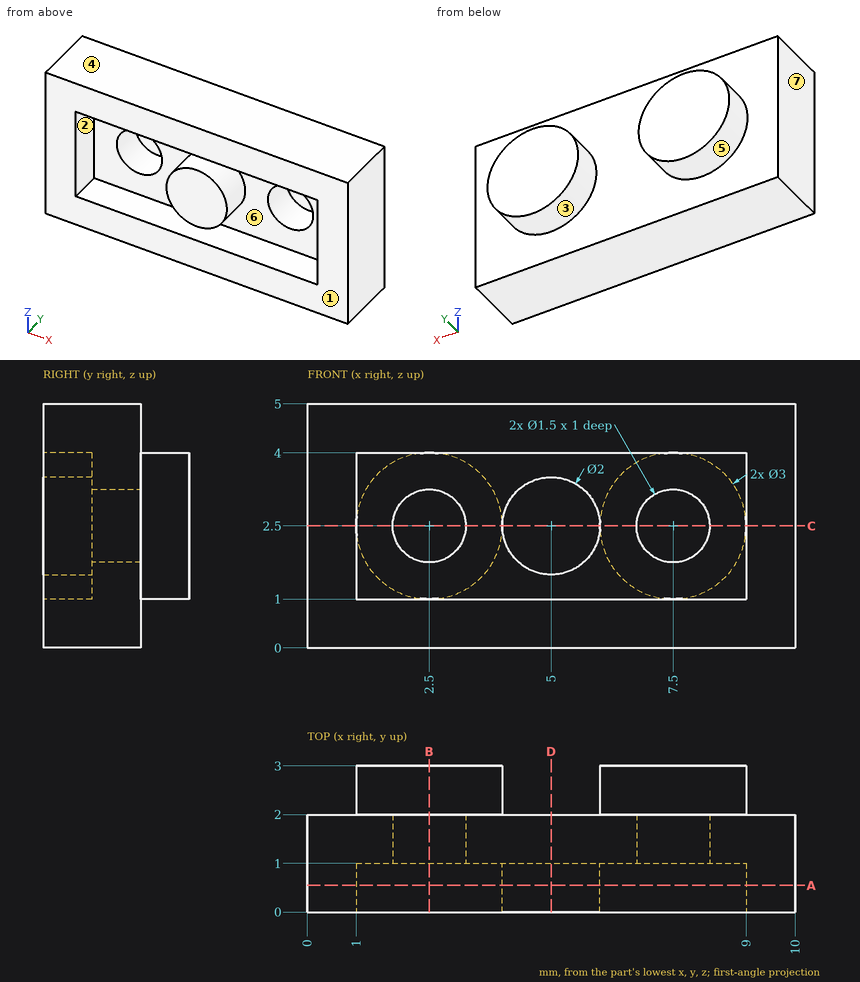
Verification items for this drawing (mm, ordinates from the low corner). A direction names the side the tool comes from. Coordinates: 2 decimals unless noted, no trailing zeros. Order: outer loops, then holes, each group sorted by start corner. A loop starts at its lowest first (then second) coordinate and runs counter-clockwise, first axis right, second up. Notation, with made-up numbers: M 4,89 L 21,89 A30 ccw 21,113 Z; hole C 59,-21 d5. An arc over 180 degrees is marked long. Answer as a JSON object with one key per item and string values.
Q1. Cross-section at B-B on x = 2.5. Record the cut outline in (y, z).
Results are:
{"outline": "M 0,0 L 2,0 L 2,1 L 3,1 L 3,4 L 2,4 L 2,5 L 0,5 L 0,4 L 1,4 L 1,3.25 L 2,3.25 L 2,1.75 L 1,1.75 L 1,1 L 0,1 Z"}
Q2. Depth check by flat-ended pin: pin 1 Ø1.5 at (x, z) = (7, 3) entering from -Y. Enter the tip coordinate at first touch or a pass-through.
Results are:
{"pin 1": "stops at y = 1"}
Q3. Cross-section at D-D on x = 5. Record the cut outline in (y, z).
Results are:
{"outline": "M 0,0 L 2,0 L 2,5 L 0,5 L 0,4 L 1,4 L 1,3.5 L 0,3.5 L 0,1.5 L 1,1.5 L 1,1 L 0,1 Z"}
Q4. Scan lines: line 1 (X direction, y = 1.65, z = 2.5); line 2 (Z direction, x = 8.5, y = 0.5); line 3 (X direction, y = 0.2, z = 3.8). Record each from-to range of solid material in increasing order.
Results are:
{"line 1": "x = 0 to 1.75, 3.25 to 6.75, 8.25 to 10", "line 2": "z = 0 to 1, 4 to 5", "line 3": "x = 0 to 1, 9 to 10"}
Q5. Release check for a two-part mould opening along Z. For the marked faces 4, 5, 6 and 7 record: released by +Z, released by -Z, zero draft, split by the parting line, or undercut.
Results are:
{"face 4": "released by +Z", "face 5": "split by the parting line", "face 6": "undercut", "face 7": "zero draft"}
Q6. Cross-section at A-A on y = 0.55. Record the cut outline in (x, z), and give its area (3 significant figures).
Results are:
{"outline": "M 0,0 L 10,0 L 10,5 L 0,5 Z; C 5,2.5 d2; hole M 1,1 L 9,1 L 9,4 L 1,4 Z", "area": "29.1 mm²"}
Q7. Cross-section at C-C on z = 2.5. Record the cut outline in (x, y).
Results are:
{"outline": "M 0,0 L 1,0 L 1,1 L 1.75,1 L 1.75,2 L 3.25,2 L 3.25,1 L 4,1 L 4,0 L 6,0 L 6,1 L 6.75,1 L 6.75,2 L 8.25,2 L 8.25,1 L 9,1 L 9,0 L 10,0 L 10,2 L 9,2 L 9,3 L 6,3 L 6,2 L 4,2 L 4,3 L 1,3 L 1,2 L 0,2 Z"}
Q8. Tool access check on the marked faces 1, 2 and 3. Record the directions out of +Z, -Z, +X, -X, +Y, -Y that give a thin tool (end or side, any length) a straight path to the whole face; none if there is none.
Results are:
{"face 1": "+Z, -Z, +X, -X, -Y", "face 2": "-Y", "face 3": "+Y"}
